Verification items for the finished model (mm, model axes). Face numbers are marked on the shaded views. A direction names the side the tool comes from. Give positions to 0.01 mm unless a question says otherwise; leave off trailing zeros. Order: outer loops, then holes, each group sorted by start corner. A loop starts at its lowest first (then second) coordinate and runs counter-clockwise, first axis right, second up.
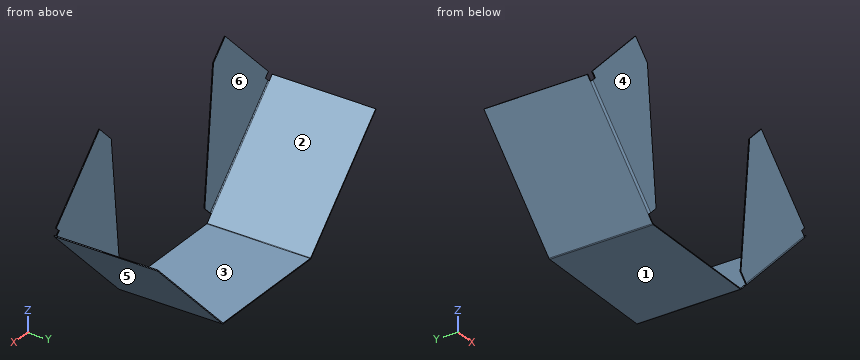
from build123d import *

# Parameters (mm, degrees)
SM_BASE_FLANGE_1_DEPTH      = 117.5
SM_EDGE_FLANGE_1_DEPTH      = 290.401572875
SM_START                    = 2
SM_EDGE_FLANGE_1_FLAT_DEPTH = 2
CUT_EXTRUDE_START           = -14
CUT_EXTRUDE_2_DEPTH         = 14


# Read off the part's stored shape, not the designer's step: 切除-拉伸2
# Sheet-metal steps are written as plain solids
with BuildPart() as part:
    # Sketch 1 → 基体-法兰1 (new, symmetric)
    with BuildSketch(Plane(origin=(0, 0, 0), x_dir=(1, 0, 0), z_dir=(0, 1, 0))):
        with BuildLine():
            Line((-367.697843509, -220.072843509), (-148.210786438, -0.585786438))
            ThreePointArc((-148.210786438, -0.585786438), (-147.56193974, -0.152240935), (-146.796572875, 0))
            Line((-146.796572875, 0), (146.796572875, 0))
            ThreePointArc((146.796572875, 0), (147.56193974, -0.152240935), (148.210786438, -0.585786438))
            Line((148.210786438, -0.585786438), (367.697843509, -220.072843509))
            Line((367.697843509, -220.072843509), (369.112057071, -218.658629946))
            Line((369.112057071, -218.658629946), (149.625, 0.828427125))
            ThreePointArc((149.625, 0.828427125), (148.327306605, 1.69551813), (146.796572875, 2))
            Line((146.796572875, 2), (-146.796572875, 2))
            ThreePointArc((-146.796572875, 2), (-148.327306605, 1.69551813), (-149.625, 0.828427125))
            Line((-149.625, 0.828427125), (-369.112057071, -218.658629946))
            Line((-369.112057071, -218.658629946), (-367.697843509, -220.072843509))
        make_face()
    extrude(amount=SM_BASE_FLANGE_1_DEPTH, both=True)

    # 边线-法兰1 bend section (across the edge) → 边线-法兰1 (add)
    with BuildSketch(Plane(origin=(162.352922061, -119.5, 14.727922061), x_dir=(0, 1, 0), z_dir=(0.7071067811865512, 0, 0.7071067811865439))):
        with BuildLine():
            Line((-2, 2), (0, 2))
            ThreePointArc((0, 2), (0.585786438, 0.585786438), (2, 0))
            Line((2, 0), (2, -2))
            ThreePointArc((2, -2), (-0.828427125, -0.828427125), (-2, 2))
        make_face()
    sm_edge_flange_1 = extrude(amount=SM_EDGE_FLANGE_1_DEPTH)

    # 边线-法兰1 profile (on flange) → 边线-法兰1 flat (add)
    with BuildSketch(Plane(origin=(73.8125, -119.5, -73.8125), x_dir=(0.7071067811865512, 0, 0.7071067811865439), z_dir=(0, -1, 0)).offset(SM_START)):
        Polygon((359.616638573, 220), (125.215065697, 27), (125.215065697, 2), (415.616638573, 2), (415.616638573, 220), align=None)
    sm_edge_flange_1_flat = extrude(amount=-SM_EDGE_FLANGE_1_FLAT_DEPTH)

    # 切除-拉伸2 outline → 切除-拉伸2 (cut)
    with BuildSketch(Plane(origin=(293.885343509, 0, 293.885343509), x_dir=(0.7071067811865338, 0, -0.7071067811865613), z_dir=(0.7071067811865613, 0, 0.7071067811865338)).offset(CUT_EXTRUDE_START)):
        with BuildLine():
            ThreePointArc((102.386638573, -121.5), (105.215065697, -120.328427125), (106.386638573, -117.5))
            Line((106.386638573, -117.5), (104.386638573, -117.5))
            ThreePointArc((104.386638573, -117.5), (103.800852135, -118.914213562), (102.386638573, -119.5))
            Line((102.386638573, -119.5), (90.386638573, -119.5))
            Line((90.386638573, -119.5), (90.386638573, -121.5))
            Line((90.386638573, -121.5), (102.386638573, -121.5))
        make_face()
    cut_extrude_2 = extrude(amount=CUT_EXTRUDE_2_DEPTH, mode=Mode.SUBTRACT)

    # 镜向1: 边线-法兰1, 边线-法兰1 flat, 切除-拉伸2 across plane
    add(sm_edge_flange_1.mirror(Plane(origin=(0, 0, 0), x_dir=(0, 0, 1), z_dir=(1, 0, 0))))
    add(sm_edge_flange_1_flat.mirror(Plane(origin=(0, 0, 0), x_dir=(0, 0, 1), z_dir=(1, 0, 0))))
    add(cut_extrude_2.mirror(Plane(origin=(0, 0, 0), x_dir=(0, 0, 1), z_dir=(1, 0, 0))), mode=Mode.SUBTRACT)


solid = part.part
(1) Set-up check for the marked faces 1, 2 and 3: record each of +Z, -Z, +X, -X, +Y, -Y from which the full face is reachable in a straight line by a thin tool's end or side.
Solved:
face 1: -Z, +X, -X, +Y, -Y
face 2: +Z, +Y
face 3: +Z, +Y, -Y
(2) Section check C-C, the plane x = 27.5. Enter the section's corners in (y, z), then the cut area to 3 significant figures.
Solved:
outline: (-117.5, -2) - (117.5, -2) - (117.5, 0) - (-117.5, 0) - close
area: 470 mm2
(3) Scan lines: line 1 (Z direction, x = -53, y = 9.5); line 2 (Y direction, x = 183.5, z = 78); line 3 (X direction, y = 92, z = 166.5) (3 decimals). Record each from-to range of solid material in increasing order.
Solved:
line 1: z = -2 to 0
line 2: y = -121.5 to -119.5
line 3: x = -316.953 to -314.125, 314.125 to 316.953
(4) Section check B-B, the plane y = 61. Enter the section's corners in (x, z) (3 decimals), then the cut area to 3 significant figures.
Solved:
outline: (-369.112, 218.659) - (-149.625, -0.828) arc R4 ccw to (-146.797, -2) - (146.797, -2) arc R4 ccw to (149.625, -0.828) - (369.112, 218.659) - (367.698, 220.073) - (148.211, 0.586) arc R2 cw to (146.797, 0) - (-146.797, 0) arc R2 cw to (-148.211, 0.586) - (-367.698, 220.073) - close
area: 1,840 mm2
(5) Go/stop test with flat-tipped pins: pin 1 (5.5 mm diameter, centred on x = 365.5, z = 216, fed in from -Y); pin 2 (5 mm diameter, centred on x = 207, z = 176, fed in from +Y); pin 3 (6 mm diameter, centred on y = 74.5, z = 59, fed in from +X). Record where each tip stops, or that it passes through.
Solved:
pin 1: stops at y = -117.5
pin 2: stops at y = -119.5
pin 3: stops at x = 212.45
(6) Section check A-A, the plane z = 248.5. Enter the section's corners in (x, y).
Solved:
outline: (-339.27, -121.5) - (-164.06, -121.5) - (-164.06, -119.5) - (-339.27, -119.5) - close; (164.06, -121.5) - (339.27, -121.5) - (339.27, -119.5) - (164.06, -119.5) - close
(7) Release check for a two-part mould opening along X. For the marked faces 4, 5 and 6 record: pulls with the +X half, pulls with the -X half, needs draft (parallel to the pull), parting line crosses it, or undercut.
Solved:
face 4: needs draft
face 5: pulls with the +X half
face 6: undercut
